The model under review builds one solid part; all positions refer to its coordinate system, in mm. A direction names the side the tool comes from. Coordinates: 2 decimals unless noted, no trailing zeros. Loops run counter-clockwise (first coordinate to the right, second up) from the corner with the lowest first, then second, coordinate; pieces in that order, holes last. Notation, with made-up numbers: (60.5, 43.25) - (92.5, 43.25) arc R19 ccw to (92.5, 65.25) - close; hole circle Ø10 at (88, 41.25). An arc over 180 degrees is marked (long way). Use a Markdown table: item, result. Add a question column.
1) Add section D-D, the plane x = 17. Give the boundary of the cut face in (y, z).
2) Add section C-C, the plane x = 6. Give the boundary of the cut face in (y, z).
3) Add section B-B, the plane z = 14.75. Give the boundary of the cut face in (x, y), and give its area (3 significant figures).
4) Add section A-A, the plane z = 3. Give the boundary of the cut face in (x, y), and give its area (3 significant figures).
5) To check wall thickness, follow L1, parallel to Y at x = 25, z = 1; L2, parallel to X at y = -14.5, z = 6.25; L3, parallel to Y at x = 38.5, z = 9. State the ranges of each line that lie inside material, in increasing order. Write a range as [from, to].
6) For faces 1 (the flat face through (25, -109, 20)), 2 (the flat face through (37.14, -15, 13)), list the 3-axis set-ups (+Z, -Z, +X, -X, +Y, -Y) from which the entire face can be reached by the end or side of a thin tool; tool diameter is ignored.
7) Clearance check with flat-ended pins moving along their axes: pin 1 (6 mm diameter, centred on y = -100, z = 14, fed in from -X); pin 2 (2 mm diameter, centred on y = -179.5, z = 13.5, fed in from +X); pin 3 (2.5 mm diameter, centred on y = -2.5, z = 16, fed in from -X). State where each tip first meets the part, or that it passes through.
8) The part is to be moulded in two halves that separate along Y. For faces 3 (the flat face through (25, -25, 13)), 4 (the flat face through (12.86, -15, 13)), 5 (the cylindrical face through (0.16, -202.16, 10.14)), say which applies: pulls with the +Y half, pulls with the -Y half, needs draft (parallel to the pull), parting line crosses it, or undercut.
```python
from build123d import *

# Parameters (mm, degrees)
SKETCH1_W           = 50
SKETCH1_H           = 220
BOSS_EXTRUDE1_DEPTH = 20
SKETCH2_R           = 2
SKETCH2_R_2         = 6
CUT_EXTRUDE2_DEPTH  = 34
FILLET2_R           = 10
CUT_EXTRUDE3_DEPTH  = 15
SKETCH7_R           = 1
CUT_EXTRUDE4_DEPTH  = 15
CUT_EXTRUDE6_DEPTH  = 15
CUT_EXTRUDE7_DEPTH  = 53


with BuildPart() as part:
    # Sketch1 → Boss-Extrude1 (new body)
    with BuildSketch(Plane.XY):
        with Locations((25, -110)):
            Rectangle(SKETCH1_W, SKETCH1_H)
    extrude(amount=BOSS_EXTRUDE1_DEPTH)

    # Sketch2 → Cut-Extrude2 (cut)
    with BuildSketch(Plane.XY.offset(20)):
        with Locations((25, -15)):
            Circle(SKETCH2_R)
        with Locations((25, -205)):
            Circle(SKETCH2_R_2)
    extrude(amount=-CUT_EXTRUDE2_DEPTH, mode=Mode.SUBTRACT)

    # Fillet2
    fillet2_edges = [part.edges().sort_by_distance(p)[0] for p in [
        (0, 0, 10),
        (50, 0, 10),
        (50, -220, 10),
        (0, -220, 10),
    ]]
    fillet(fillet2_edges, radius=FILLET2_R)

    # Sketch4 → Cut-Extrude3 (cut)
    with BuildSketch(Plane.XY.offset(20)):
        Polygon((25, -25), (37.14, -25), (37.14, 0), (12.86, 0), (12.86, -25), align=None)
    extrude(amount=-CUT_EXTRUDE3_DEPTH, mode=Mode.SUBTRACT)

    # Sketch7 → Cut-Extrude4 (cut)
    with BuildSketch(Plane(origin=(0, 0, 0), x_dir=(-1, 0, 0), z_dir=(0, 0, -1))):
        with Locations((-25, -10.5)):
            Circle(SKETCH7_R)
        with Locations((-25, -19.5)):
            Circle(SKETCH7_R)
    extrude(amount=-CUT_EXTRUDE4_DEPTH, mode=Mode.SUBTRACT)

    # Sketch8 → Cut-Extrude6 (cut)
    with BuildSketch(Plane.XY.offset(20)):
        with BuildLine():
            Line((12.86, -4.956404509), (37.14, -4.956404509))
            Line((37.14, -4.956404509), (37.14, 0))
            Line((37.14, 0), (40, 0))
            ThreePointArc((40, 0), (40.933059212, -0.043625132), (41.857977457, -0.174119899))
            Line((41.857977457, -0.174119899), (41.857977457, 3.191267917))
            Line((41.857977457, 3.191267917), (8.577977457, 3.191267917))
            Line((8.577977457, 3.191267917), (8.577977457, -0.101623775))
            ThreePointArc((8.577977457, -0.101623775), (9.287175424, -0.025438299), (10, 0))
            Line((10, 0), (12.86, 0))
            Line((12.86, 0), (12.86, -4.956404509))
        make_face()
        with BuildLine():
            Line((8.577977457, -4.956404509), (12.86, -4.956404509))
            Line((12.86, -4.956404509), (12.86, 0))
            Line((12.86, 0), (10, 0))
            ThreePointArc((10, 0), (9.287175424, -0.025438299), (8.577977457, -0.101623775))
            Line((8.577977457, -0.101623775), (8.577977457, -4.956404509))
        make_face()
        with BuildLine():
            Line((37.14, 0), (37.14, -4.956404509))
            Line((37.14, -4.956404509), (41.857977457, -4.956404509))
            Line((41.857977457, -4.956404509), (41.857977457, -0.174119899))
            ThreePointArc((41.857977457, -0.174119899), (40.933059212, -0.043625132), (40, 0))
            Line((40, 0), (37.14, 0))
        make_face()
    extrude(amount=-CUT_EXTRUDE6_DEPTH, mode=Mode.SUBTRACT)

    # Sketch9 → Cut-Extrude7 (cut)
    with BuildSketch(Plane.XY.offset(20)):
        with BuildLine():
            ThreePointArc((49.336156478, -199.277108434), (49.833484572, -202.119367426), (50, -205))
            Line((50, -205), (50, -202.054385429))
            Line((50, -202.054385429), (50, -15))
            ThreePointArc((50, -15), (49.833484572, -17.880632574), (49.336156478, -20.722891566))
            ThreePointArc((49.336156478, -20.722891566), (38.980197534, -110), (49.336156478, -199.277108434))
        make_face()
        with BuildLine():
            Line((0, -19.137020496), (0, -205))
            ThreePointArc((0, -205), (0.166515428, -202.119367426), (0.663843522, -199.277108434))
            ThreePointArc((0.663843522, -199.277108434), (11.019802466, -110), (0.663843522, -20.722891566))
            ThreePointArc((0.663843522, -20.722891566), (0.166515428, -17.880632574), (0, -15))
            Line((0, -15), (0, -19.137020496))
        make_face()
    extrude(amount=-CUT_EXTRUDE7_DEPTH, mode=Mode.SUBTRACT)


solid = part.part
```
From the geometry:
| question | item | result |
|---|---|---|
| 1 | outline | (-220, 0) - (0, 0) - (0, 5) - (-25, 5) - (-25, 20) - (-220, 20) - close |
| 2 | outline | (-219.17, 0) - (-172.37, 0) - (-172.37, 20) - (-219.17, 20) - close; (-47.63, 0) - (-0.83, 0) - (-0.83, 20) - (-47.63, 20) - close |
| 3 | outline | (0, -210) arc R10 ccw to (10, -220) - (40, -220) arc R10 ccw to (50, -210) - (50, -205) arc R25 ccw to (49.34, -199.28) arc R390 cw to (49.34, -20.72) arc R25 ccw to (50, -15) - (50, -10) arc R10 ccw to (41.86, -0.17) - (41.86, -4.96) - (37.14, -4.96) - (37.14, -25) - (12.86, -25) - (12.86, -4.96) - (8.58, -4.96) - (8.58, -0.1) arc R10 ccw to (0, -10) - (0, -15) arc R25 ccw to (0.66, -20.72) arc R390 cw to (0.66, -199.28) arc R25 ccw to (0, -205) - close; hole circle Ø12 at (25, -205) |
| 3 | area | 7,440 mm^2 |
| 4 | outline | (0, -210) arc R10 ccw to (10, -220) - (40, -220) arc R10 ccw to (50, -210) - (50, -205) arc R25 ccw to (49.34, -199.28) arc R390 cw to (49.34, -20.72) arc R25 ccw to (50, -15) - (50, -10) arc R10 ccw to (40, 0) - (10, 0) arc R10 ccw to (0, -10) - (0, -15) arc R25 ccw to (0.66, -20.72) arc R390 cw to (0.66, -199.28) arc R25 ccw to (0, -205) - close; hole circle Ø12 at (25, -205); hole circle Ø4 at (25, -15); hole circle Ø2 at (25, -19.5); hole circle Ø2 at (25, -10.5) |
| 4 | area | 8,070 mm^2 |
| 5 | L1 | y = [-220, -211], [-199, -20.5], [-18.5, -17], [-13, -11.5], [-9.5, 0] |
| 5 | L2 | x = [0, 12.86], [37.14, 50] |
| 5 | L3 | y = [-220, -4.96] |
| 6 | face 1 | +Z, +X, -X, +Y, -Y |
| 6 | face 2 | +Z, +Y |
| 7 | pin 1 | stops at x = 10.8 |
| 7 | pin 2 | stops at x = 45.41 |
| 7 | pin 3 | stops at x = 2.19 |
| 8 | face 3 | pulls with the +Y half |
| 8 | face 4 | needs draft |
| 8 | face 5 | undercut |
